Source: CAD feature listing. Evaluate the final solid. Frame: model axes, mm. Face numbers are marked on the shaded views. A direction names the side the tool comes from. Give positions to 0.01 mm unless a question says otherwise; leave off trailing zeros. Order: outer loops, then holes, each group sorted by start corner. A loop starts at its lowest first (then second) coordinate and runs counter-clockwise, first axis right, second up. Notation, with made-up numbers: (-27, 20) -> (27, 20) arc R19 cw to (27, 26) -> close; hole circle Ø2 at (21.25, -21). An arc over 180 degrees is marked (long way). Answer in a Markdown table with one row per item.
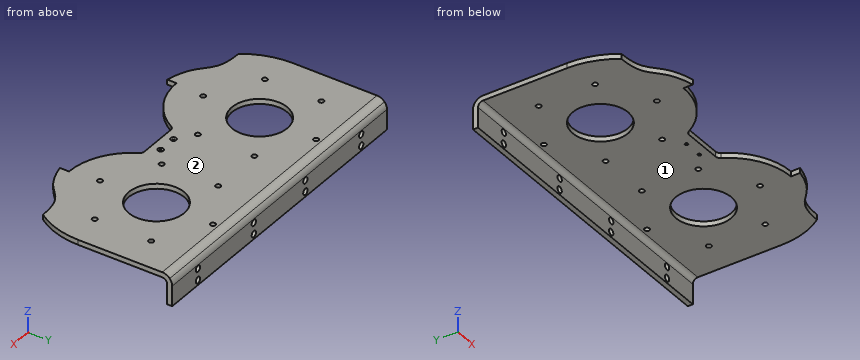
```python
from build123d import *

# Parameters (mm, degrees)
SKETCH1_W                                           = 250
SKETCH1_H                                           = 155.2734375
BOSS_EXTRUDE1_DEPTH                                 = 4
FILLET1_R                                           = 62.5
CUT_EXTRUDE1_DEPTH                                  = 10
CUT_EXTRUDE2_DEPTH                                  = 10
SKETCH7_R                                           = 22
CUT_EXTRUDE3_DEPTH                                  = 7
SKETCH8_W                                           = 250
SKETCH8_H                                           = 19.85691045
CUT_EXTRUDE4_DEPTH                                  = 7
BOSS_EXTRUDE6_DEPTH                                 = 250
CUT_EXTRUDE6_DEPTH                                  = 250
CIRPATTERN1_COUNT                                   = 6
F_5_0_5_DIAMETER_HOLE2_AT_2_COUNT                   = 2
F_5_0_5_DIAMETER_HOLE2_AT_2_PITCH                   = 9
LPATTERN2_COUNT                                     = 2
LPATTERN2_PITCH                                     = 65
CSK_FOR_M2_COUNTERSUNK_FLAT_HEAD_SCREW1_D           = 2.4
CSK_FOR_M2_COUNTERSUNK_FLAT_HEAD_SCREW1_DEPTH       = 9
CSK_FOR_M2_COUNTERSUNK_FLAT_HEAD_SCREW1_CSINK_D     = 4.4
CSK_FOR_M2_COUNTERSUNK_FLAT_HEAD_SCREW1_CSINK_ANGLE = 90
CSK_FOR_M2_COUNTERSUNK_FLAT_HEAD_SCREW1_TIP         = 0.721032743


with BuildPart() as part:
    # Sketch1 → Boss-Extrude1 (new body)
    with BuildSketch(Plane.XY):
        with Locations((0, -2.7798083)):
            Rectangle(SKETCH1_W, SKETCH1_H)
    extrude(amount=BOSS_EXTRUDE1_DEPTH)

    # Fillet1
    fillet1_edges = [part.edges().sort_by_distance(p)[0] for p in [
        (125, -80.41652705, 2),
        (-125, -80.41652705, 2),
    ]]
    fillet(fillet1_edges, radius=FILLET1_R)

    # Sketch5 → Cut-Extrude1 (cut)
    with BuildSketch(Plane.XY.offset(4)):
        with BuildLine():
            Line((15.296531701, -40.14308955), (-15.296531701, -40.14308955))
            ThreePointArc((-15.296531701, -40.14308955), (-17.324975275, -40.695566285), (-18.793084909, -42.200381217))
            ThreePointArc((-18.793084909, -42.200381217), (-37.144455324, -61.01056787), (-62.5, -67.91652705))
            Line((-62.5, -67.91652705), (-62.5, -80.41652705))
            Line((-62.5, -80.41652705), (62.5, -80.41652705))
            Line((62.5, -80.41652705), (62.5, -67.91652705))
            ThreePointArc((62.5, -67.91652705), (37.144455324, -61.01056787), (18.793084909, -42.200381217))
            ThreePointArc((18.793084909, -42.200381217), (17.324975275, -40.695566285), (15.296531701, -40.14308955))
        make_face()
    extrude(amount=-CUT_EXTRUDE1_DEPTH, mode=Mode.SUBTRACT)

    # Sketch6 → Cut-Extrude2 (cut)
    with BuildSketch(Plane.XY.offset(4)):
        with BuildLine():
            Line((-113.871867123, -53.514016685), (-113.871867123, -84.736307966))
            Line((-113.871867123, -84.736307966), (-44.821444402, -84.736307966))
            Line((-44.821444402, -84.736307966), (-44.821444402, -77.864159797))
            add(Edge.make_bspline(
                [(-113.871867123, -53.514016685), (-77.935103041, -53.525535165), (-98.515305829, -73.080146865), (-44.821444402, -77.864159797)],
                knots=[0, 0, 0, 0, 1, 1, 1, 1], degree=3))
        make_face()
    cut_extrude2 = extrude(amount=-CUT_EXTRUDE2_DEPTH, mode=Mode.SUBTRACT)

    # Mirror2: Cut-Extrude2 across plane
    add(cut_extrude2.mirror(Plane(origin=(0, 0, 0), x_dir=(0, 0, 1), z_dir=(1, 0, 0))), mode=Mode.SUBTRACT)

    # Sketch7 → Cut-Extrude3 (cut)
    with BuildSketch(Plane.XY.offset(4)):
        with Locations((-60, 0)):
            Circle(SKETCH7_R)
    cut_extrude3 = extrude(amount=-CUT_EXTRUDE3_DEPTH, mode=Mode.SUBTRACT)

    # Mirror3: Cut-Extrude3 across plane
    add(cut_extrude3.mirror(Plane(origin=(0, 0, 0), x_dir=(0, 0, 1), z_dir=(1, 0, 0))), mode=Mode.SUBTRACT)

    # Sketch8 → Cut-Extrude4 (cut)
    with BuildSketch(Plane.XY.offset(4)):
        with Locations((0, 64.928455225)):
            Rectangle(SKETCH8_W, SKETCH8_H)
    extrude(amount=-CUT_EXTRUDE4_DEPTH, mode=Mode.SUBTRACT)

    # Sketch20 → Boss-Extrude6 (add)
    with BuildSketch(Plane.ZY.offset(125)):
        with BuildLine():
            Line((4, 45.281624312), (0, 45.281624312))
            Line((0, 45.281624312), (0, 49.00347295))
            ThreePointArc((0, 49.00347295), (-1.171572875, 51.831900074), (-4, 53.00347295))
            Line((-4, 53.00347295), (-20, 53.00347295))
            Line((-20, 53.00347295), (-20, 57.00347295))
            Line((-20, 57.00347295), (-4, 57.00347295))
            ThreePointArc((-4, 57.00347295), (1.656854249, 54.660327199), (4, 49.00347295))
            Line((4, 49.00347295), (4, 45.281624312))
        make_face()
    extrude(amount=-BOSS_EXTRUDE6_DEPTH)

    # Sketch22 → Cut-Extrude6 (cut)
    with BuildSketch(Plane.ZY.offset(125)):
        with BuildLine():
            Line((1.295437974, 55), (4, 55))
            Line((4, 55), (4, 49.00347295))
            ThreePointArc((4, 49.00347295), (3.292581977, 52.292583484), (1.295437974, 55))
        make_face()
    extrude(amount=-CUT_EXTRUDE6_DEPTH, mode=Mode.SUBTRACT)

    # Sketch3 → Ø4.0mm Dowel Hole1 (revolve, cut)
    with BuildSketch(Plane(origin=(-60, 45, 4), x_dir=(0, -1, 0), z_dir=(1, 0, 0))):
        Polygon((0, 0), (0, 51.201721238), (2, 50), (2, 0), align=None)
    f_4_0mm_dowel_hole1 = revolve(axis=Axis((-60, 45, 10.35), (0, 0, -1)), mode=Mode.SUBTRACT)

    # CirPattern1: Ø4.0mm Dowel Hole1 ×6 about axis
    cirpattern1_axis = Axis((-60, 0, 0), (0, 0, 1))
    for i in range(1, CIRPATTERN1_COUNT):
        add(f_4_0mm_dowel_hole1.rotate(cirpattern1_axis, i * 360 / CIRPATTERN1_COUNT), mode=Mode.SUBTRACT)

    # Mirror1: Ø4.0mm Dowel Hole1 across plane
    add(f_4_0mm_dowel_hole1.mirror(Plane(origin=(0, 0, 0), x_dir=(0, 0, 1), z_dir=(1, 0, 0))), mode=Mode.SUBTRACT)

    # Mirror1 copy 1 sketch → Mirror1 copy 1 (revolve, cut)
    with BuildSketch(Plane(origin=(98.97114317, 22.5, 4), x_dir=(-0.8660254037844386, -0.5000000000000001, 0), z_dir=(-0.5000000000000001, 0.8660254037844386, 0))):
        Polygon((0, 0), (0, -51.201721238), (2, -50), (2, 0), align=None)
    revolve(axis=Axis((98.97114317, 22.5, 10.35), (0, 0, 1)), mode=Mode.SUBTRACT)

    # Mirror1 copy 2 sketch → Mirror1 copy 2 (revolve, cut)
    with BuildSketch(Plane(origin=(98.97114317, -22.5, 4), x_dir=(-0.8660254037844387, 0.4999999999999998, 0), z_dir=(0.4999999999999998, 0.8660254037844387, 0))):
        Polygon((0, 0), (0, -51.201721238), (2, -50), (2, 0), align=None)
    revolve(axis=Axis((98.97114317, -22.5, 10.35), (0, 0, 1)), mode=Mode.SUBTRACT)

    # Mirror1 copy 3 sketch → Mirror1 copy 3 (revolve, cut)
    with BuildSketch(Plane(origin=(60, -45, 4), x_dir=(0, 1, 0), z_dir=(1, 0, 0))):
        Polygon((0, 0), (0, -51.201721238), (2, -50), (2, 0), align=None)
    revolve(axis=Axis((60, -45, 10.35), (0, 0, 1)), mode=Mode.SUBTRACT)

    # Mirror1 copy 4 sketch → Mirror1 copy 4 (revolve, cut)
    with BuildSketch(Plane(origin=(21.02885683, -22.5, 4), x_dir=(0.8660254037844384, 0.5000000000000004, 0), z_dir=(0.5000000000000004, -0.8660254037844384, 0))):
        Polygon((0, 0), (0, -51.201721238), (2, -50), (2, 0), align=None)
    revolve(axis=Axis((21.02885683, -22.5, 10.35), (0, 0, 1)), mode=Mode.SUBTRACT)

    # Mirror1 copy 5 sketch → Mirror1 copy 5 (revolve, cut)
    with BuildSketch(Plane(origin=(21.02885683, 22.5, 4), x_dir=(0.8660254037844386, -0.5000000000000001, 0), z_dir=(-0.5000000000000001, -0.8660254037844386, 0))):
        Polygon((0, 0), (0, -51.201721238), (2, -50), (2, 0), align=None)
    revolve(axis=Axis((21.02885683, 22.5, 10.35), (0, 0, 1)), mode=Mode.SUBTRACT)

    # Sketch24 → Ø5.0 (5) Diameter Hole2 (revolve, cut)
    with BuildSketch(Plane(origin=(-95, 57.00347295, -16), x_dir=(0, 0, 1), z_dir=(1, 0, 0))):
        Polygon((0, 0), (0, 51.502151548), (2.5, 50), (2.5, 0), align=None)
    f_5_0_5_diameter_hole2 = revolve(axis=Axis((-95, 63.35347295, -16), (0, -1, 0)), mode=Mode.SUBTRACT)

    # Ø5.0 (5) Diameter Hole2 at 2: Ø5.0 (5) Diameter Hole2 ×2
    with Locations(*[(0, 0, i * F_5_0_5_DIAMETER_HOLE2_AT_2_PITCH) for i in range(1, F_5_0_5_DIAMETER_HOLE2_AT_2_COUNT)]):
        add(f_5_0_5_diameter_hole2, mode=Mode.SUBTRACT)

    # LPattern2: Ø5.0 (5) Diameter Hole2 ×2
    with Locations(*[(i * LPATTERN2_PITCH, 0, 0) for i in range(1, LPATTERN2_COUNT)]):
        add(f_5_0_5_diameter_hole2, mode=Mode.SUBTRACT)

    # LPattern2 copy 1 sketch → LPattern2 copy 1 (revolve, cut)
    with BuildSketch(Plane(origin=(-30, 57.00347295, -7), x_dir=(0, 0, 1), z_dir=(1, 0, 0))):
        Polygon((0, 0), (0, 51.502151548), (2.5, 50), (2.5, 0), align=None)
    revolve(axis=Axis((-30, 63.35347295, -7), (0, -1, 0)), mode=Mode.SUBTRACT)

    # Mirror6: Ø5.0 (5) Diameter Hole2 across plane
    add(f_5_0_5_diameter_hole2.mirror(Plane(origin=(0, 0, 0), x_dir=(0, 0, 1), z_dir=(1, 0, 0))), mode=Mode.SUBTRACT)

    # Mirror6 copy 1 sketch → Mirror6 copy 1 (revolve, cut)
    with BuildSketch(Plane(origin=(95, 57.00347295, -7), x_dir=(0, 0, 1), z_dir=(-1, 0, 0))):
        Polygon((0, 0), (0, -51.502151548), (2.5, -50), (2.5, 0), align=None)
    revolve(axis=Axis((95, 63.35347295, -7), (0, 1, 0)), mode=Mode.SUBTRACT)

    # Mirror6 copy 2 sketch → Mirror6 copy 2 (revolve, cut)
    with BuildSketch(Plane(origin=(30, 57.00347295, -16), x_dir=(0, 0, 1), z_dir=(-1, 0, 0))):
        Polygon((0, 0), (0, -51.502151548), (2.5, -50), (2.5, 0), align=None)
    revolve(axis=Axis((30, 63.35347295, -16), (0, 1, 0)), mode=Mode.SUBTRACT)

    # Mirror6 copy 3 sketch → Mirror6 copy 3 (revolve, cut)
    with BuildSketch(Plane(origin=(30, 57.00347295, -7), x_dir=(0, 0, 1), z_dir=(-1, 0, 0))):
        Polygon((0, 0), (0, -51.502151548), (2.5, -50), (2.5, 0), align=None)
    revolve(axis=Axis((30, 63.35347295, -7), (0, 1, 0)), mode=Mode.SUBTRACT)

    # CSK for M2 Countersunk Flat Head Screw1
    with Locations(Plane.XY.offset(4)):
        with Locations((-7.5, -32.64308955), (7.5, -32.64308955)):
            CounterSinkHole(CSK_FOR_M2_COUNTERSUNK_FLAT_HEAD_SCREW1_D / 2, CSK_FOR_M2_COUNTERSUNK_FLAT_HEAD_SCREW1_CSINK_D / 2, depth=CSK_FOR_M2_COUNTERSUNK_FLAT_HEAD_SCREW1_DEPTH, counter_sink_angle=CSK_FOR_M2_COUNTERSUNK_FLAT_HEAD_SCREW1_CSINK_ANGLE)
            with Locations((0, 0, -(CSK_FOR_M2_COUNTERSUNK_FLAT_HEAD_SCREW1_DEPTH + CSK_FOR_M2_COUNTERSUNK_FLAT_HEAD_SCREW1_TIP / 2))):  # 118° drill point
                Cone(0, CSK_FOR_M2_COUNTERSUNK_FLAT_HEAD_SCREW1_D / 2, CSK_FOR_M2_COUNTERSUNK_FLAT_HEAD_SCREW1_TIP, mode=Mode.SUBTRACT)


solid = part.part
```
(1) Section query C-C (x = 30). Return the cut outline in (y, z), plus the area to 3 significant figures.
A:
| item | result |
|---|---|
| outline | (-55.91, 0) -> (49, 0) arc R4 cw to (53, -4) -> (53, -4.5) -> (57, -4.5) -> (57, -4) arc R8 ccw to (49, 4) -> (-55.91, 4) -> close; (53, -20) -> (57, -20) -> (57, -18.5) -> (53, -18.5) -> close; (53, -13.5) -> (57, -13.5) -> (57, -9.5) -> (53, -9.5) -> close |
| area | 481 mm^2 |
(2) Section query B-B (y = 18). Return the cut outline in (x, z).
A:
| item | result |
|---|---|
| outline | (-125, 0) -> (-72.65, 0) -> (-72.65, 4) -> (-125, 4) -> close; (-47.35, 0) -> (47.35, 0) -> (47.35, 4) -> (-47.35, 4) -> close; (72.65, 0) -> (125, 0) -> (125, 4) -> (72.65, 4) -> close |
(3) Access query for the marked faces 1 and 2. Directions: +Z, -Z, +X, -X, +Y, -Y. A direction counts if a zero-diameter tool reaches every point of the face in a straight line with its end or side. Return the directions, or none.
A:
| item | result |
|---|---|
| face 1 | -Z, +X, -X, -Y |
| face 2 | +Z, +X, -X, +Y, -Y |
(4) Section query A-A (z = -7). Return the cut outline in (x, y).
A:
| item | result |
|---|---|
| outline | (-125, 53) -> (-97.5, 53) -> (-97.5, 57) -> (-125, 57) -> close; (-92.5, 53) -> (-32.5, 53) -> (-32.5, 57) -> (-92.5, 57) -> close; (-27.5, 53) -> (27.5, 53) -> (27.5, 57) -> (-27.5, 57) -> close; (32.5, 53) -> (92.5, 53) -> (92.5, 57) -> (32.5, 57) -> close; (97.5, 53) -> (125, 53) -> (125, 57) -> (97.5, 57) -> close |
(5) First-contact query: pin 1 Ø13 at (x, z) = (-34, -13) entering from -Y; pin 2 Ø5 at (x, y) = (98, 19) entering from -Z; pin 3 Ø4 at (x, z) = (95, -7) entering from -Y; pin 4 Ø6.5 at (x, z) = (30, -16) entering from +Y. Flat tips, straight axial feed; report the tip coordinate or a pass-through.
A:
| item | result |
|---|---|
| pin 1 | stops at y = 53 |
| pin 2 | stops at z = 0 |
| pin 3 | passes through |
| pin 4 | stops at y = 57 |
(6) Ray query, probe 1 along X at (y, z) = (54.65, -7); probe 2 along Z at (x, y) = (-85.5, -26); probe 3 along Y at (x, z) = (-107.5, -7.75). Return the intervals inside material, ascending.
A:
| item | result |
|---|---|
| probe 1 | x = -125 to -97.5, -92.5 to -32.5, -27.5 to 27.5, 32.5 to 92.5, 97.5 to 125 |
| probe 2 | z = 0 to 4 |
| probe 3 | y = 53 to 57 |
